from build123d import *

# Parameters (mm, degrees)
SKETCH1_W                                           = 140
SKETCH1_H                                           = 65
BOSS_EXTRUDE1_DEPTH                                 = 15
SKETCH2_R                                           = 15
SKETCH2_R_2                                         = 2.5
CUT_EXTRUDE2_DEPTH                                  = 27
TAP_DRILL_FOR_M6_TAP1_D                             = 5
TAP_DRILL_FOR_M6_TAP1_DEPTH                         = 15
TAP_DRILL_FOR_M6_TAP1_TIP                           = 1.502151548
CBORE_FOR_M6_HEX_SOCKET_HEAD_CAP_SCREW3_D           = 6.6
CBORE_FOR_M6_HEX_SOCKET_HEAD_CAP_SCREW3_CBORE_D     = 11
CBORE_FOR_M6_HEX_SOCKET_HEAD_CAP_SCREW3_CBORE_DEPTH = 61.4
SKETCH29_W                                          = 35
SKETCH29_H                                          = 2
CUT_EXTRUDE6_DEPTH                                  = 79.620925968
CHAMFER2_SIZE                                       = 10
SKETCH30_R                                          = 20
CUT_EXTRUDE7_DEPTH                                  = 4


with BuildPart() as part:
    # Sketch1 → Boss-Extrude1 (new body)
    with BuildSketch(Plane.XY):
        Rectangle(SKETCH1_W, SKETCH1_H)
    extrude(amount=BOSS_EXTRUDE1_DEPTH)

    # Sketch2 → Cut-Extrude2 (cut)
    with BuildSketch(Plane(origin=(0, 0, 15), x_dir=(-1, 0, 0), z_dir=(0, 0, -1))):
        with Locations(Location((0, -2.5, 0), (0, 0, 180))):
            Circle(SKETCH2_R)
        with Locations(Location((-23.57, 21.07, 0), (0, 0, 180))):
            Circle(SKETCH2_R_2)
        with Locations(Location((23.57, 21.07, 0), (0, 0, 180))):
            Circle(SKETCH2_R_2)
        with Locations(Location((23.57, -26.07, 0), (0, 0, 180))):
            Circle(SKETCH2_R_2)
        with Locations(Location((-23.57, -26.07, 0), (0, 0, 180))):
            Circle(SKETCH2_R_2)
    extrude(amount=CUT_EXTRUDE2_DEPTH, mode=Mode.SUBTRACT)

    # Tap Drill for M6 Tap1
    with Locations(Plane(origin=(70, 0, 0), x_dir=(0, 0, -1), z_dir=(1, 0, 0))):
        with Locations((-7.5, -17.5)):
            Hole(TAP_DRILL_FOR_M6_TAP1_D / 2, depth=TAP_DRILL_FOR_M6_TAP1_DEPTH)
            with Locations((0, 0, -(TAP_DRILL_FOR_M6_TAP1_DEPTH + TAP_DRILL_FOR_M6_TAP1_TIP / 2))):  # 118° drill point
                Cone(0, TAP_DRILL_FOR_M6_TAP1_D / 2, TAP_DRILL_FOR_M6_TAP1_TIP, mode=Mode.SUBTRACT)

    # CBORE for M6 Hex Socket Head Cap Screw3 (through all)
    with Locations(Plane(origin=(0, 32.5, 0), x_dir=(1, 0, 0), z_dir=(0, 1, 0))):
        with Locations((40, -7.5), (-40, -7.5)):
            CounterBoreHole(CBORE_FOR_M6_HEX_SOCKET_HEAD_CAP_SCREW3_D / 2, CBORE_FOR_M6_HEX_SOCKET_HEAD_CAP_SCREW3_CBORE_D / 2, CBORE_FOR_M6_HEX_SOCKET_HEAD_CAP_SCREW3_CBORE_DEPTH)

    # Sketch29 → Cut-Extrude6 (cut, through all)
    with BuildSketch(Plane.XY.offset(15)):
        with Locations((0, -31.5)):
            Rectangle(SKETCH29_W, SKETCH29_H)
    extrude(amount=-CUT_EXTRUDE6_DEPTH, mode=Mode.SUBTRACT)

    # Chamfer2
    # the kernel refuses this chamfer: 10 mm, written as the material it adds along each edge
    with BuildSketch(Plane(origin=(-17.5, -30.5, 15), x_dir=(-0.027495876610591493, -0.9996219169112965, 0), z_dir=(0, 0, -1))) as chamfer2_piece_1_section:
        Polygon((CHAMFER2_SIZE * 0.999621916911, -CHAMFER2_SIZE * 0.0274958766106), (-CHAMFER2_SIZE * 0.0274958766106, -CHAMFER2_SIZE * 0.999621916911), (0, 0), align=None)
    chamfer2_piece_1 = extrude(amount=15, mode=Mode.PRIVATE)
    chamfer2_piece_1 = split(chamfer2_piece_1, bisect_by=Plane(origin=(-12.880949734, -32.5, 7.5), z_dir=(0, 1, 0)), keep=Keep.TOP, mode=Mode.PRIVATE)
    add(chamfer2_piece_1)
    with BuildSketch(Plane(origin=(17.5, -30.5, 15), x_dir=(-0.9996219169112968, 0.027495876610586317, 0), z_dir=(0, 0, -1))) as chamfer2_piece_2_section:
        Polygon((CHAMFER2_SIZE * 0.999621916911, -CHAMFER2_SIZE * 0.0274958766106), (-CHAMFER2_SIZE * 0.0274958766106, -CHAMFER2_SIZE * 0.999621916911), (0, 0), align=None)
    chamfer2_piece_2 = extrude(amount=15, mode=Mode.PRIVATE)
    chamfer2_piece_2 = split(chamfer2_piece_2, bisect_by=Plane(origin=(12.880949734, -32.5, 7.5), z_dir=(0, 1, 0)), keep=Keep.TOP, mode=Mode.PRIVATE)
    add(chamfer2_piece_2)

    # Sketch30 → Cut-Extrude7 (cut)
    with BuildSketch(Plane(origin=(0, 0, 0), x_dir=(-1, 0, 0), z_dir=(0, 0, -1))):
        with Locations((0, -2.5)):
            Circle(SKETCH30_R)
    extrude(amount=-CUT_EXTRUDE7_DEPTH, mode=Mode.SUBTRACT)


solid = part.part
Input: part model. Units: mm. Frame: model coordinates. A direction names the side the tool comes from. Coordinates: 2 decimals unless noted, no trailing zeros. Loops run counter-clockwise (first coordinate to the right, second up) from the corner with the lowest first, then second, coordinate; pieces in that order, holes last.
Q1. Cut plane A-A (x = -40). Output: boundary loops of the cut face in (y, z), then the cut area to 3 significant figures.
Q2. Cut plane D-D (x = 23.57). Output: boundary loops of the cut face in (y, z), then the cut area to 3 significant figures.
Q3. Material intervals for line 1 (Y direction, x = -23.57, z = 6.25); line 2 (X direction, y = -26.07, z = 5.5); line 3 (X direction, y = 27, z = 3.25), sorted ascending.
Q4. Cut plane C-C (y = 21.07). Output: boundary loops of the cut face in (x, z).
Q5. Set-up query: faces 1 (the face through (35.6, 2.2, 10.8)), 2 (the face through (21.73, -27.76, 7.6)), 3 (the face through (-2.9, 12.4, 4)), 4 (the face through (0, -30.5, 8)). Return all of +Z, -Z, +X, -X, +Y, -Y with unobstructed straight access to the full face (end or side cutting, diameter ignored); none if empty.
Q6. Draft query along X for faces 5 (the face through (-1, 32.5, 7)), 6 (the face through (53.759, -17.481, 7.934)), 7 (the face through (-3.252, 12.143, 9.577)). Return one class per face: +X half, -X half, draft (parallel to the pull), parting line (faces both ways), or undercut.
Q7. Cut plane B-B (y = -2.5). Output: boundary loops of the cut face in (x, z).
Q8. Contact query for flat-ended pins moving along their axis: pin 1 (4 mm diameter, centred on x = -6, z = 8.5, fed in from -Y); pin 2 (4 mm diameter, centred on x = -40, z = 7.5, fed in from +Y); pin 3 (5.5 mm diameter, centred on x = 42.5, z = 9.5, fed in from +Y). Output: stop coordinate, or through.
Working result:
1. outline: (-32.5, 0) - (32.5, 0) - (32.5, 2) - (-28.9, 2) - (-28.9, 4.2) - (-32.5, 4.2) - close; (-32.5, 10.8) - (-28.9, 10.8) - (-28.9, 13) - (32.5, 13) - (32.5, 15) - (-32.5, 15) - close
1. area: 276 mm2
2. outline: (-32.5, 0) - (-28.57, 0) - (-28.57, 15) - (-32.5, 15) - close; (-23.57, 0) - (18.57, 0) - (18.57, 15) - (-23.57, 15) - close; (23.57, 0) - (32.5, 0) - (32.5, 15) - (23.57, 15) - close
2. area: 825 mm2
3. line 1: y = -32.5 to -28.57, -23.57 to 18.57, 23.57 to 32.5
3. line 2: x = -70 to -45.12, -34.88 to -26.07, -21.07 to 21.07, 26.07 to 34.88, 45.12 to 70
3. line 3: x = -70 to -43.49, -36.51 to 36.51, 43.49 to 70
4. outline: (-70, 0) - (-26.07, 0) - (-26.07, 15) - (-70, 15) - close; (-21.07, 0) - (21.07, 0) - (21.07, 15) - (-21.07, 15) - close; (26.07, 0) - (70, 0) - (70, 15) - (26.07, 15) - close; hole circle Ø11 at (-40, 7.5); hole circle Ø11 at (40, 7.5)
5. face 1: +Y
5. face 2: +Z, -Z
5. face 3: -Z
5. face 4: +Z, -Z, -Y
6. face 5: draft
6. face 6: +X half
6. face 7: undercut
7. outline: (-70, 0) - (-20, 0) - (-20, 4) - (-15, 4) - (-15, 15) - (-70, 15) - close; (15, 4) - (20, 4) - (20, 0) - (70, 0) - (70, 15) - (15, 15) - close; hole circle Ø11 at (-40, 7.5); hole circle Ø11 at (40, 7.5)
8. pin 1: stops at y = -31
8. pin 2: passes through
8. pin 3: stops at y = 32.5
